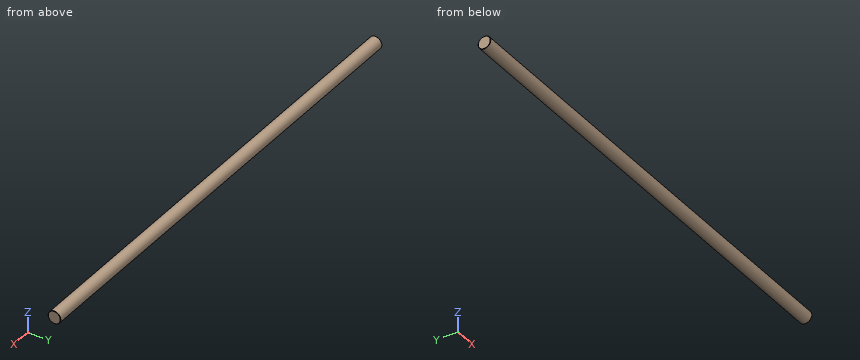
```python
from build123d import *

# Parameters (mm, degrees)
SKETCH1_R           = 4
BOSS_EXTRUDE1_DEPTH = 300
SKETCH5_OUTSIDE_W   = 672.15
SKETCH5_OUTSIDE_H   = 672.15
SKETCH5_OUTSIDE_R   = 3.8
CUT_EXTRUDE2_DEPTH  = 301.053328593
CUT_EXTRUDE2_DRAFT  = -45
SKETCH6_OUTSIDE_W   = 672.15
SKETCH6_OUTSIDE_H   = 672.15
SKETCH6_OUTSIDE_R   = 3.8
CUT_EXTRUDE3_DEPTH  = 301.053328593
CUT_EXTRUDE3_DRAFT  = -45


with BuildPart() as part:
    # Sketch1 → Boss-Extrude1 (new body)
    with BuildSketch(Plane(origin=(0, 0, 0), x_dir=(0, 0, -1), z_dir=(1, 0, 0))):
        Circle(SKETCH1_R)
    extrude(amount=BOSS_EXTRUDE1_DEPTH)


with BuildPart() as cut_extrude2_tool:
    # Sketch5 outside → Cut-Extrude2 (with draft: the straight prism first)
    with BuildSketch(Plane.ZY):
        Rectangle(SKETCH5_OUTSIDE_W, SKETCH5_OUTSIDE_H)
        Circle(SKETCH5_OUTSIDE_R, mode=Mode.SUBTRACT)
    extrude(amount=-CUT_EXTRUDE2_DEPTH)
    # Cut-Extrude2: the draft: its side faces are tilted about the plane it starts from
    cut_extrude2_sides = [cut_extrude2_tool.faces().sort_by_distance(p)[0] for p in [
        (150.526664297, -336.075, 0),
        (150.526664297, 0, 336.075),
        (150.526664297, 336.075, 0),
        (150.526664297, 0, -336.075),
        (150.526664297, 0, -3.8),
    ]]
    draft(cut_extrude2_sides, Plane.ZY, CUT_EXTRUDE2_DRAFT)


with BuildPart() as part_1:
    add(part.part)

    # Cut-Extrude2: cut by cut_extrude2_tool
    add(cut_extrude2_tool.part, mode=Mode.SUBTRACT)


with BuildPart() as cut_extrude3_tool:
    # Sketch6 outside → Cut-Extrude3 (with draft: the straight prism first)
    with BuildSketch(Plane(origin=(300, 0, 0), x_dir=(0, 0, -1), z_dir=(1, 0, 0))):
        Rectangle(SKETCH6_OUTSIDE_W, SKETCH6_OUTSIDE_H)
        Circle(SKETCH6_OUTSIDE_R, mode=Mode.SUBTRACT)
    extrude(amount=-CUT_EXTRUDE3_DEPTH)
    # Cut-Extrude3: the draft: its side faces are tilted about the plane it starts from
    cut_extrude3_sides = [cut_extrude3_tool.faces().sort_by_distance(p)[0] for p in [
        (149.473335703, -336.075, 0),
        (149.473335703, 0, -336.075),
        (149.473335703, 336.075, 0),
        (149.473335703, 0, 336.075),
        (149.473335703, 0, 3.8),
    ]]
    draft(cut_extrude3_sides, Plane(origin=(300, 0, 0), x_dir=(0, 0, -1), z_dir=(1, 0, 0)), CUT_EXTRUDE3_DRAFT)


with BuildPart() as part_2:
    add(part_1.part)

    # Cut-Extrude3: cut by cut_extrude3_tool
    add(cut_extrude3_tool.part, mode=Mode.SUBTRACT)


solid = part_2.part
```
Input: part model. Units: mm. Frame: model coordinates. Coordinates: 2 decimals unless noted, no trailing zeros. Write each loop counter-clockwise with the first axis right and the second up, starting at its lowest first coordinate (ties: lowest second). Pieces come first, ordered by that corner, then holes.
1) Section A-A on x = 35. Output: boundary loops of the cut face in (y, z), and give its area (3 significant figures).
2) Material intervals for line 1 along Z through (x, y) = (180.5, 0.25); line 2 along Z through (x, y) = (35.5, -1.25); line 3 along Y through (x, z) = (96, 3.5), sorted ascending.
3) Pin query (flat end, axial travel): pin 1 Ø2 at (x, y) = (152, 2.5) entering from -Z; pin 2 Ø2 at (x, z) = (210.5, -2.5) entering from +Y. Return the tip coordinate at first contact, or that it passes through.
Check result:
1. outline: circle Ø8 at (0, 0)
1. area: 50.3 mm2
2. line 1: z = -3.99 to 3.99
2. line 2: z = -3.8 to 3.8
2. line 3: y = -1.94 to 1.94
3. pin 1: stops at z = -3.71
3. pin 2: stops at y = 3.71
